```python
from build123d import *

# Parameters (mm, degrees)
SKETCH1_R                     = 28.829
SKETCH1_R_2                   = 7.9375
BOSS_EXTRUDE1_DEPTH           = 3.175
TAP_DRILL_FOR_4_40_TAP1_D     = 2.2606
TAP_DRILL_FOR_4_40_TAP1_DEPTH = 4
TAP_DRILL_FOR_4_40_TAP1_TIP   = 0.679152758


with BuildPart() as part:
    # Sketch1 → Boss-Extrude1 (new body)
    with BuildSketch(Plane.XY):
        Circle(SKETCH1_R)
        Circle(SKETCH1_R_2, mode=Mode.SUBTRACT)
    extrude(amount=BOSS_EXTRUDE1_DEPTH)

    # Tap Drill for #4-40 Tap1
    with Locations(Plane.XY.offset(3.175)):
        with Locations((0, 12.7), (0, -12.7), (12.7, 0), (-12.7, 0)):
            Hole(TAP_DRILL_FOR_4_40_TAP1_D / 2, depth=TAP_DRILL_FOR_4_40_TAP1_DEPTH)
            with Locations((0, 0, -(TAP_DRILL_FOR_4_40_TAP1_DEPTH + TAP_DRILL_FOR_4_40_TAP1_TIP / 2))):  # 118° drill point
                Cone(0, TAP_DRILL_FOR_4_40_TAP1_D / 2, TAP_DRILL_FOR_4_40_TAP1_TIP, mode=Mode.SUBTRACT)


solid = part.part
```
Could you check a few things on this model? Use its own coordinates, in mm. Round coordinates to 2 decimals unless told otherwise and drop trailing zeros. Loops run counter-clockwise (first coordinate to the right, second up) from the corner with the lowest first, then second, coordinate; pieces in that order, holes last. Notation, with made-up numbers: (11.5, -39.5) -> (45.5, -39.5) arc R29 ccw to (45.5, -18.5) -> close; hole circle Ø1 at (-36, -34.75). An arc over 180 degrees is marked (long way). One line per question, with ' | ' between items.
(1) For pin 1 Ø1.5 at (y, z) = (-10.5, 2.5) entering from +X, with a flat end and sliding along its axis, tell me the tip position at first contact or that it passes through.
Model answer:
pin 1: stops at x = 27.13
(2) If we section it at D-D on y = -19.5: List the corners of the cut face in (x, z) for me (1 decimal).
Model answer:
outline: (-21.2, 0) -> (21.2, 0) -> (21.2, 3.2) -> (-21.2, 3.2) -> close
(3) If we section it at A-A on y = 6.5: List the corners of the cut face in (x, z) for me (3 decimals).
Model answer:
outline: (-28.087, 0) -> (-4.556, 0) -> (-4.556, 3.175) -> (-28.087, 3.175) -> close; (4.556, 0) -> (28.087, 0) -> (28.087, 3.175) -> (4.556, 3.175) -> close
(4) If we section it at B-B on x = 12.7: List the corners of the cut face in (y, z) for me (3 decimals), and give its area (3 significant figures).
Model answer:
outline: (-25.881, 0) -> (-1.13, 0) -> (-1.13, 3.175) -> (-25.881, 3.175) -> close; (1.13, 0) -> (25.881, 0) -> (25.881, 3.175) -> (1.13, 3.175) -> close | area: 157 mm^2
(5) If I drill on probe 1 along Y at (x, z) = (0, 1.75); probe 2 along Y at (x, z) = (4, 1.4); probe 3 along Y at (x, z) = (-5.5, 0.65), over which ranges is the centre line in solid material (lowest first)?
Model answer:
probe 1: y = -28.83 to -13.83, -11.57 to -7.94, 7.94 to 11.57, 13.83 to 28.83 | probe 2: y = -28.55 to -6.86, 6.86 to 28.55 | probe 3: y = -28.3 to -5.72, 5.72 to 28.3
(6) Thinking about a two-plate mould opening in Y: for faces 1 (the face through (-11.9, 0.8, 1.6)), 2 (the face through (6, -6, 0)), 3 (the face through (-6.25, -28.143, 1.565)), which applies, released by +Y, released by -Y, zero draft, split by the parting line, or undercut?
Model answer:
face 1: undercut | face 2: zero draft | face 3: split by the parting line
(7) If we section it at C-C on z = 1.3: List the corners of the cut face in (x, y) for me (1 decimal), and give its area (3 significant figures).
Model answer:
outline: circle Ø57.7 at (0, 0); hole circle Ø2.3 at (-12.7, 0); hole circle Ø15.9 at (0, 0); hole circle Ø2.3 at (0, -12.7); hole circle Ø2.3 at (0, 12.7); hole circle Ø2.3 at (12.7, 0) | area: 2,400 mm^2
